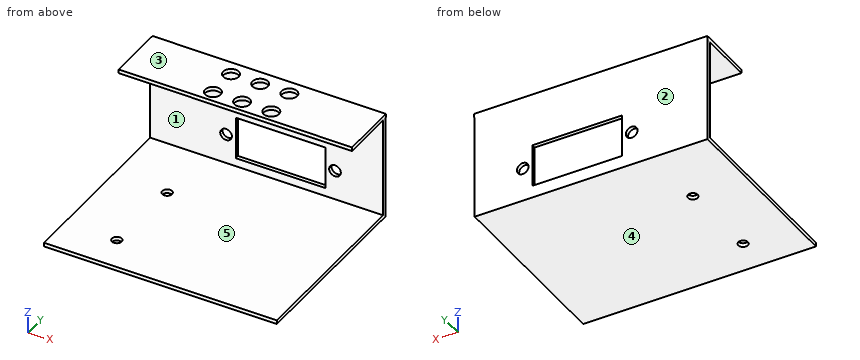
from build123d import *

# Parameters (mm, degrees)
ESQUISSE1_W             = 60
ESQUISSE1_H             = 15
BOSS_EXTRU_1_DEPTH      = 1
ESQUISSE2_W             = 59.836868209
ESQUISSE2_H             = 27
BOSS_EXTRU_2_DEPTH      = 1
ESQUISSE4_W             = 59.836868209
ESQUISSE4_H             = 47
BOSS_EXTRU_3_DEPTH      = 1
ESQUISSE6_R             = 2
ENL_V_MAT_EXTRU_5_DEPTH = 1
ESQUISSE8_W             = 23
ESQUISSE8_H             = 11
ENL_V_MAT_EXTRU_7_DEPTH = 1
ESQUISSE9_R             = 1.5
ENL_V_MAT_EXTRU_8_DEPTH = 1
ESQUISSE10_R            = 1.25
ENL_V_MAT_EXTRU_9_DEPTH = 1


with BuildPart() as part:
    # Esquisse1 → Boss.-Extru.1 (new body)
    with BuildSketch(Plane.XY):
        Rectangle(ESQUISSE1_W, ESQUISSE1_H)
    extrude(amount=BOSS_EXTRU_1_DEPTH)

    # Esquisse2 → Boss.-Extru.2 (add)
    with BuildSketch(Plane(origin=(0, 7.5, 0), x_dir=(1, 0, 0), z_dir=(0, 1, 0))):
        with Locations((-0.085609374, 13.5)):
            Rectangle(ESQUISSE2_W, ESQUISSE2_H)
    extrude(amount=-BOSS_EXTRU_2_DEPTH)

    # Esquisse4 → Boss.-Extru.3 (add)
    with BuildSketch(Plane.XY.offset(-27)):
        with Locations((-0.085609374, -17)):
            Rectangle(ESQUISSE4_W, ESQUISSE4_H)
    extrude(amount=BOSS_EXTRU_3_DEPTH)

    # Esquisse6 → Enlèv. mat.-Extru.5 (cut)
    with BuildSketch(Plane.XY.offset(1)):
        with Locations((-7.5, 3.5)):
            Circle(ESQUISSE6_R)
        with Locations((0, 3.5)):
            Circle(ESQUISSE6_R)
        with Locations((7.5, 3.5)):
            Circle(ESQUISSE6_R)
        with Locations(Location((7.5, -4.5, 0), (0, 0, 180))):
            Circle(ESQUISSE6_R)
        with Locations(Location((0, -4.5, 0), (0, 0, 180))):
            Circle(ESQUISSE6_R)
        with Locations(Location((-7.5, -4.5, 0), (0, 0, 180))):
            Circle(ESQUISSE6_R)
    extrude(amount=-ENL_V_MAT_EXTRU_5_DEPTH, mode=Mode.SUBTRACT)

    # Esquisse8 → Enlèv. mat.-Extru.7 (cut)
    with BuildSketch(Plane(origin=(0, 7.5, 0), x_dir=(1, 0, 0), z_dir=(0, 1, 0))):
        with Locations((3.484076767, 18.307447957)):
            Rectangle(ESQUISSE8_W, ESQUISSE8_H)
    extrude(amount=-ENL_V_MAT_EXTRU_7_DEPTH, mode=Mode.SUBTRACT)

    # Esquisse9 → Enlèv. mat.-Extru.8 (cut)
    with BuildSketch(Plane(origin=(0, 7.5, 0), x_dir=(1, 0, 0), z_dir=(0, 1, 0))):
        with Locations(Location((17.484076767, 18.264970918, 0), (0, 0, 180))):
            Circle(ESQUISSE9_R)
        with Locations(Location((-10.515923233, 18.264970918, 0), (0, 0, 180))):
            Circle(ESQUISSE9_R)
    extrude(amount=-ENL_V_MAT_EXTRU_8_DEPTH, mode=Mode.SUBTRACT)

    # Esquisse10 → Enlèv. mat.-Extru.9 (cut)
    with BuildSketch(Plane(origin=(0, 0, -27), x_dir=(-1, 0, 0), z_dir=(0, 0, -1))):
        with Locations((16.528262126, -31.490674341)):
            Circle(ESQUISSE10_R)
        with Locations((16.074327743, -9.995466885)):
            Circle(ESQUISSE10_R)
    extrude(amount=-ENL_V_MAT_EXTRU_9_DEPTH, mode=Mode.SUBTRACT)


solid = part.part
For this review, take the finished solid that the model builds, in its own axes (mm). Face numbers are marked on the shaded views. A direction names the side the tool comes from. Round coordinates to 2 decimals unless told otherwise and drop trailing zeros. Order: outer loops, then holes, each group sorted by start corner. A loop starts at its lowest first (then second) coordinate and runs counter-clockwise, first axis right, second up. Notation, with made-up numbers: (-27.5, 53.25) -> (22.5, 53.25) arc R18 ccw to (22.5, 76.25) -> close; hole circle Ø2 at (7, -9.5). An arc over 180 degrees is marked (long way). Put each result on its own line as item: value.
Q1. For probe 1 along Y at (x, z) = (-7.5, 0.5); probe 2 along X at (y, z) = (-4.5, 0.65); probe 3 along Z at (x, y) = (18, -3), list the stretches that pass through material, from the lowest coordinate up. Write a range as [from, to].
Check result:
probe 1: [-7.5, -6.5], [-2.5, 1.5], [5.5, 7.5]
probe 2: [-30, -9.5], [-5.5, -2], [2, 5.5], [9.5, 30]
probe 3: [-27, -26], [0, 1]
Q2. Mouldability with a two-part tool opening along Z and no side actions: class the marked faces 3, 4 and 5 as pulls with the +Z half, pulls with the -Z half, needs draft (parallel to the pull), parting line crosses it, or undercut.
Check result:
face 3: pulls with the +Z half
face 4: pulls with the -Z half
face 5: undercut
Q3. Machinability: for the marked faces 1 and 2, which of the approach directions +Z, -Z, +X, -X, +Y, -Y give a long, thin tool a straight path to every point of the face, cutting with its end or side? Answer none if there is none.
Check result:
face 1: +X, -X, -Y
face 2: +Z, -Z, +X, -X, +Y
Q4. Add section B-B on y = 3.5. Write out the cut boundary in (x, z), plus the area to 3 significant figures.
Check result:
outline: (-30, -27) -> (29.83, -27) -> (29.83, -26) -> (-30, -26) -> close; (-30, 0) -> (-9.5, 0) -> (-9.5, 1) -> (-30, 1) -> close; (-5.5, 0) -> (-2, 0) -> (-2, 1) -> (-5.5, 1) -> close; (2, 0) -> (5.5, 0) -> (5.5, 1) -> (2, 1) -> close; (9.5, 0) -> (30, 0) -> (30, 1) -> (9.5, 1) -> close
area: 108 mm2
Q5. Add section A-A on x = 3.5. Write out the cut boundary in (y, z).
Check result:
outline: (-40.5, -27) -> (7.5, -27) -> (7.5, -23.81) -> (6.5, -23.81) -> (6.5, -26) -> (-40.5, -26) -> close; (-7.5, 0) -> (6.5, 0) -> (6.5, -12.81) -> (7.5, -12.81) -> (7.5, 1) -> (-7.5, 1) -> close
Q6. Insertion check: pin 1 Ø6.5 at (x, y) = (0, -4.5) entering from +Z; pin 2 Ø2 at (x, z) = (4.5, -15) entering from +Y; pin 3 Ø0.8 at (x, z) = (-14, 0.5) entering from -Y; pin 4 Ø4 at (x, y) = (7, -30) entering from +Z. Each pin has a flat end and moves straight along its axis. Give the tip position at first contact, or say it passes through.
Check result:
pin 1: z = 1
pin 2: through
pin 3: y = -7.5
pin 4: z = -26
Q7. Add section C-C on x = 26.5. Write out the cut boundary in (y, z).
Check result:
outline: (-40.5, -27) -> (7.5, -27) -> (7.5, 1) -> (-7.5, 1) -> (-7.5, 0) -> (6.5, 0) -> (6.5, -26) -> (-40.5, -26) -> close
Q8. Add section D-D on y = -12. Write out the cut boundary in (x, z), plus the area to 3 significant figures.
Check result:
outline: (-30, -27) -> (29.83, -27) -> (29.83, -26) -> (-30, -26) -> close
area: 59.8 mm2
